```python
from build123d import *

# Parameters (mm, degrees)
BOSS_EXTRUDE1_DEPTH      = 80
BOSS_EXTRUDE2_DEPTH      = 25
SKETCH5_W                = 100
SKETCH5_H                = 2
BOSS_EXTRUDE3_DEPTH      = 1
BOSS_EXTRUDE3_DEPTH_BACK = 69
CUT_EXTRUDE1_DEPTH       = 54
CUT_EXTRUDE1_DEPTH_BACK  = 128
BOSS_EXTRUDE4_DEPTH      = 80
BOSS_EXTRUDE5_DEPTH      = 2
BOSS_EXTRUDE6_DEPTH      = 2
CUT_EXTRUDE2_DEPTH       = 10
SKETCH12_W               = 66.626507626
SKETCH12_H               = 2
BOSS_EXTRUDE7_DEPTH      = 3
SKETCH13_W               = 64.876762197
SKETCH13_H               = 2
BOSS_EXTRUDE8_DEPTH      = 3
CUT_EXTRUDE3_DEPTH       = 61.618605692


with BuildPart() as part:
    # Sketch1 → Boss-Extrude1 (new body)
    with BuildSketch(Plane.XY):
        Polygon((33.482657766, -45.251477229), (33.482657766, -66.768484939), (-31.394104431, -66.768484939), (-31.394104431, -53.768484939), (-54.654934222, -68.768484939), (35.482657766, -68.768484939), (35.482657766, -43.768484939), (-24.517342234, -43.768484939), (-24.517342234, -28.768484939), (-64.517342234, -28.768484939), (-64.517342234, -68.768484939), (-62.012951809, -68.768484939), (-62.012951809, -63.171810384), (-27.383124188, -45.251477229), align=None)
    extrude(amount=BOSS_EXTRUDE1_DEPTH)

    # Sketch4 → Boss-Extrude2 (add)
    with BuildSketch(Plane(origin=(0, -43.768484939, 0), x_dir=(1, 0, 0), z_dir=(0, 1, 0))):
        Polygon((-54.654934222, -80), (-31.394104431, -80), (-31.394104431, -55), align=None)
        Polygon((-54.654934222, 0), (-31.394104431, 0), (-31.394104431, -25), align=None)
    extrude(amount=-BOSS_EXTRUDE2_DEPTH)

    # Sketch5 → Boss-Extrude3 (add, two sides)
    with BuildSketch(Plane(origin=(0, 0, 0), x_dir=(1, 0, 0), z_dir=(0, 1, 0))) as boss_extrude3_sk:
        with Locations((-14.517342234, -79)):
            Rectangle(SKETCH5_W, SKETCH5_H)
        with Locations((-14.517342234, -1)):
            Rectangle(SKETCH5_W, SKETCH5_H)
    extrude(amount=BOSS_EXTRUDE3_DEPTH)
    extrude(boss_extrude3_sk.sketch, amount=-BOSS_EXTRUDE3_DEPTH_BACK)

    # Sketch6 → Cut-Extrude1 (cut, two sides)
    with BuildSketch(Plane(origin=(0, 0, 0), x_dir=(-1, 0, 0), z_dir=(0, 0, -1))) as cut_extrude1_sk:
        Polygon((64.517342234, -28.768484939), (24.517342234, -28.768484939), (24.517342234, -43.768484939), (-35.482657766, -43.768484939), (-64.959998335, 15.691238157), (80.820060582, 20.703322698), align=None)
    extrude(amount=CUT_EXTRUDE1_DEPTH, mode=Mode.SUBTRACT)
    extrude(cut_extrude1_sk.sketch, amount=-CUT_EXTRUDE1_DEPTH_BACK, mode=Mode.SUBTRACT)

    # Sketch7 → Boss-Extrude4 (add)
    with BuildSketch(Plane.XY.offset(80)):
        Polygon((-40.942007341, -69), (-55.024396115, -69), (-62.814493255, -74), align=None)
        Polygon((-47.280486214, -68.008659762), (-52.794067838, -67.568484939), (-55.024396115, -69), (-40.942007341, -69), (-39.368534116, -68.640307638), align=None)
    extrude(amount=-BOSS_EXTRUDE4_DEPTH)

    # Sketch9 → Boss-Extrude5 (add)
    with BuildSketch(Plane.XY.offset(80)):
        Polygon((-64.517342234, -69), (-55.024396115, -69), (-62.814493255, -74), align=None)
    extrude(amount=-BOSS_EXTRUDE5_DEPTH)

    # Sketch10 → Boss-Extrude6 (add)
    with BuildSketch(Plane(origin=(0, 0, 0), x_dir=(-1, 0, 0), z_dir=(0, 0, -1))):
        Polygon((64.517342234, -69), (55.024396115, -69), (62.814493255, -74), align=None)
    extrude(amount=-BOSS_EXTRUDE6_DEPTH)

    # Sketch11 → Cut-Extrude2 (cut)
    with BuildSketch(Plane(origin=(0, -43.768484939, 0), x_dir=(1, 0, 0), z_dir=(0, 1, 0))):
        with BuildLine():
            ThreePointArc((-17.017342234, -40), (5.482657766, -62.5), (27.982657766, -40))
            Line((27.982657766, -40), (-17.017342234, -40))
        make_face()
        with BuildLine():
            Line((-17.017342234, -40), (27.982657766, -40))
            ThreePointArc((27.982657766, -40), (5.482657766, -17.5), (-17.017342234, -40))
        make_face()
    extrude(amount=-CUT_EXTRUDE2_DEPTH, mode=Mode.SUBTRACT)

    # Sketch12 → Boss-Extrude7 (add)
    with BuildSketch(Plane(origin=(0, 0, 78), x_dir=(-1, 0, 0), z_dir=(0, 0, -1))):
        with Locations((-1.919149382, -64.768484939)):
            Rectangle(SKETCH12_W, SKETCH12_H)
    extrude(amount=BOSS_EXTRUDE7_DEPTH)

    # Sketch13 → Boss-Extrude8 (add)
    with BuildSketch(Plane.XY.offset(2)):
        with Locations((1.044276668, -64.768484939)):
            Rectangle(SKETCH13_W, SKETCH13_H)
    extrude(amount=BOSS_EXTRUDE8_DEPTH)

    # Sketch14 → Cut-Extrude3 (cut)
    with BuildSketch(Plane(origin=(35.482657766, 0, 0), x_dir=(0, 0, -1), z_dir=(1, 0, 0))):
        Polygon((-2, -65.768484939), (-78, -65.768484939), (-78, -66.768484939), (-71.1896289, -66.768484939), (-71.1896289, -68.768484939), (-40, -68.768484939), (-8.8103711, -68.768484939), (-8.8103711, -66.768484939), (-2, -66.768484939), align=None)
    extrude(amount=-CUT_EXTRUDE3_DEPTH, mode=Mode.SUBTRACT)


solid = part.part
```
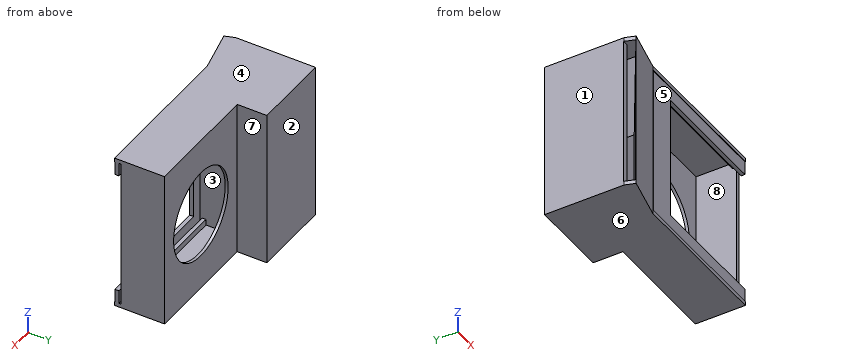
Verification items for the finished model (mm, model axes). Face numbers are marked on the shaded views. A direction names the side the tool comes from. Round coordinates to 2 decimals unless told otherwise and drop trailing zeros. Write each loop counter-clockwise with the first axis right and the second up, starting at its lowest first coordinate (ties: lowest second). Pieces come first, ordered by that corner, then holes. Notation, with made-up numbers: (71, -12.75) -> (96, -12.75) arc R29 cw to (96, 7.25) -> close; hole circle Ø10 at (-18.5, 0). An arc over 180 degrees is marked (long way). Write each question's results on one line, items separated by ' | '.
Q1. Sectioned sample at C-C, the plane x = 2. Record the boundary of the cut face in (y, z), and give its area (3 significant figures).
Derived:
outline: (-69, 0) -> (-43.77, 0) -> (-43.77, 17.77) -> (-45.25, 17.77) -> (-45.25, 2) -> (-63.77, 2) -> (-63.77, 5) -> (-65.77, 5) -> (-65.77, 2) -> (-66.77, 2) -> (-66.77, 8.81) -> (-68.77, 8.81) -> (-68.77, 2) -> (-69, 2) -> close; (-69, 78) -> (-68.77, 78) -> (-68.77, 71.19) -> (-66.77, 71.19) -> (-66.77, 78) -> (-65.77, 78) -> (-65.77, 75) -> (-63.77, 75) -> (-63.77, 78) -> (-45.25, 78) -> (-45.25, 62.23) -> (-43.77, 62.23) -> (-43.77, 80) -> (-69, 80) -> close | area: 187 mm²
Q2. Sectioned sample at B-B, the plane y = -56. Record the boundary of the cut face in (x, z).
Derived:
outline: (-64.52, 0) -> (35.48, 0) -> (35.48, 80) -> (-64.52, 80) -> close; hole (-48.15, 6.99) -> (-34.85, 21.28) -> (-34.85, 58.72) -> (-48.15, 73.01) -> close; hole (-31.39, 2) -> (33.48, 2) -> (33.48, 78) -> (-31.39, 78) -> close
Q3. Go/stop test with flat-tipped pins: pin 1 Ø12 at (y, z) = (-33, 47) entering from +X; pin 2 Ø8 at (x, y) = (2, -65.5) entering from -Z; pin 3 Ø0.9 at (x, z) = (-11, 3) entering from +Y; pin 4 Ø20 at (x, z) = (9.5, 49.5) entering from -Y. Record where each tip stops, or that it passes through.
Derived:
pin 1: stops at x = -24.52 | pin 2: stops at z = 0 | pin 3: stops at y = -43.77 | pin 4: passes through
Q4. Sectioned sample at D-D, the plane z = 58. Record the boundary of the cut face in (x, y).
Derived:
outline: (-64.52, -68.77) -> (-62.01, -68.77) -> (-62.01, -63.17) -> (-34.19, -48.77) -> (-34.19, -55.57) -> (-52.79, -67.57) -> (-62.81, -74) -> (-39.93, -68.77) -> (-26.14, -68.77) -> (-26.14, -66.77) -> (-31.39, -66.77) -> (-31.39, -47.33) -> (-27.38, -45.25) -> (-8.02, -45.25) -> (-8.02, -43.77) -> (-24.52, -43.77) -> (-24.52, -28.77) -> (-64.52, -28.77) -> close; (18.98, -45.25) -> (33.48, -45.25) -> (33.48, -65.77) -> (35.48, -65.77) -> (35.48, -43.77) -> (18.98, -43.77) -> close
Q5. Thickness scan on probe 1 along Y at (x, z) = (-3, 76.5); probe 2 along X at (y, z) = (-44, 40); probe 3 along Z at (x, y) = (1, -54). Record the ranges inside material, lowest first.
Derived:
probe 1: y = -68.77 to -66.77, -65.77 to -63.77, -45.25 to -43.77 | probe 2: x = -64.52 to -17.02, 27.98 to 35.48 | probe 3: z = 0 to 2, 78 to 80
Q6. Access from +Z, -Z, +X, -X, +Y, -Y to the whole of each face (thin tool, end or side, straight path). Record for the marked faces 4, 5, 6, 7 and 8.
Derived:
face 4: +Z, +X, -X, +Y, -Y | face 5: +X, -Y | face 6: -Z, +X, -X, +Y, -Y | face 7: +Z, -Z, +X, +Y | face 8: none
Q7. Draft check along X on the marked faces 1, 2 and 3. Enter one of: released by +X, released by -X, zero draft, split by the parting line, or undercut.
Derived:
face 1: released by -X | face 2: zero draft | face 3: undercut
Q8. Sectioned sample at A-A, the plane z = 40. Record the boundary of the cut face in (x, y), and give its area (3 significant figures).
Derived:
outline: (-64.52, -68.77) -> (-62.01, -68.77) -> (-62.01, -63.17) -> (-27.38, -45.25) -> (-17.02, -45.25) -> (-17.02, -43.77) -> (-24.52, -43.77) -> (-24.52, -28.77) -> (-64.52, -28.77) -> close; (-62.81, -74) -> (-39.93, -68.77) -> (-26.14, -68.77) -> (-26.14, -66.77) -> (-31.39, -66.77) -> (-31.39, -53.77) -> (-52.79, -67.57) -> close; (27.98, -45.25) -> (33.48, -45.25) -> (33.48, -65.77) -> (35.48, -65.77) -> (35.48, -43.77) -> (27.98, -43.77) -> close | area: 1,320 mm²
